The listing builds one solid part. Answer for the finished solid, in the listing's coordinates (mm). A direction names the side the tool comes from. Give positions to 0.01 mm unless a question says otherwise; leave off trailing zeros. Loops run counter-clockwise (first coordinate to the right, second up) from the corner with the lowest first, then second, coordinate; pieces in that order, holes last. Notation, with made-up numbers: M -8.75,83 L 29.25,83 A34 ccw 29.25,113 Z; hole C 40,15.25 d8. An arc over 180 degrees is marked long. One line per item, written item: value. Start each with the question number.
Q1. For faces 4 (the flat face through (39, 3, 35)), 5 (the cylindrical face through (-43.103, 2.958, 31.21)), 6 (the flat face through (-40, 3, 35)), determine the directions among +Z, -Z, +X, -X, +Y, -Y from which every point of the face is accessible in a straight line to the end or side of a thin tool.
Q2. The mould has two halves that part along Z. Classify faces 1 (the flat face through (-39, 3, -35)), 2 (the cylindrical face through (0, 3, 44)), 3 (the cylindrical face through (-0.469, 2.958, 47.498)): +Z half, -Z half, draft (parallel to the pull), parting line (faces both ways), or undercut.
Q3. Flat-ended cylindrical pins translate along their axes: pin 1 (3 mm diameter, centred on x = -37.5, y = 4, fed in from -Z); pin 2 (3 mm diameter, centred on x = -40.5, y = 4.5, fed in from +Z); pin 3 (1.5 mm diameter, centred on x = 21.5, y = 2.5, fed in from -Z). Find the tip coordinate at first contact, or state that the pin passes through.
Q4. Consider L1, parallel to X at y = 2.75, z = 0; L2, parallel to X at y = 4, z = 30; L3, parallel to Z at x = -42.5, y = 3.85. Determine where each line is inside the solid, lowest interval first.
Q5. A cutting plane is placed at C-C, the plane y = 3.5. State how many separate pieces and enclosed holes the cut face has, and give its area (3 significant figures).
Q6. A cutting plane is placed at D-D, the plane x = -17. Determine the outline of the cut face in (y, z), and give its area (3 significant figures).
Q7. A cutting plane is placed at A-A, the plane x = 0. Determine the outline of the cut face in (y, z).
Q8. A cutting plane is placed at B-B, the plane z = 12. Determine the outline of the cut face in (x, y), and give its area (3 significant figures).
from build123d import *

# Parameters (mm, degrees)
SKETCH1_R           = 2.25
SKETCH1_R_2         = 25
SKETCH1_R_3         = 1.5
BOSS_EXTRUDE1_DEPTH = 6


with BuildPart() as part:
    # Sketch1 → Boss-Extrude1 (new body)
    with BuildSketch(Plane(origin=(0, 0, 0), x_dir=(1, 0, 0), z_dir=(0, 1, 0))):
        with BuildLine():
            Line((50, -30), (50, 30))
            ThreePointArc((50, 30), (48.535533906, 33.535533906), (45, 35))
            Line((45, 35), (34.003676272, 35))
            ThreePointArc((34.003676272, 35), (32.278512373, 35.307046823), (30.765230913, 36.19047619))
            ThreePointArc((30.765230913, 36.19047619), (0, 47.5), (-30.765230913, 36.19047619))
            ThreePointArc((-30.765230913, 36.19047619), (-32.278512373, 35.307046823), (-34.003676272, 35))
            Line((-34.003676272, 35), (-45, 35))
            ThreePointArc((-45, 35), (-48.535533906, 33.535533906), (-50, 30))
            Line((-50, 30), (-50, -30))
            ThreePointArc((-50, -30), (-48.535533906, -33.535533906), (-45, -35))
            Line((-45, -35), (-34.003676272, -35))
            ThreePointArc((-34.003676272, -35), (-32.278512373, -35.307046823), (-30.765230913, -36.19047619))
            ThreePointArc((-30.765230913, -36.19047619), (0, -47.5), (30.765230913, -36.19047619))
            ThreePointArc((30.765230913, -36.19047619), (32.278512373, -35.307046823), (34.003676272, -35))
            Line((34.003676272, -35), (45, -35))
            ThreePointArc((45, -35), (48.535533906, -33.535533906), (50, -30))
        make_face()
        with Locations(Location((-45, 30, 0), (0, 0, 270))):
            Circle(SKETCH1_R, mode=Mode.SUBTRACT)
        with Locations(Location((-45, -30, 0), (0, 0, 270))):
            Circle(SKETCH1_R, mode=Mode.SUBTRACT)
        with Locations(Location((45, -30, 0), (0, 0, 270))):
            Circle(SKETCH1_R, mode=Mode.SUBTRACT)
        with Locations(Location((45, 30, 0), (0, 0, 270))):
            Circle(SKETCH1_R, mode=Mode.SUBTRACT)
        with Locations(Location((0, 0, 0), (0, 0, 270))):
            Circle(SKETCH1_R_2, mode=Mode.SUBTRACT)
        with Locations(Location((0, 42.5, 0), (0, 0, 270))):
            Circle(SKETCH1_R_3, mode=Mode.SUBTRACT)
        with Locations(Location((42.5, 0, 0), (0, 0, 270))):
            Circle(SKETCH1_R_3, mode=Mode.SUBTRACT)
        with Locations(Location((0, -42.5, 0), (0, 0, 90))):
            Circle(SKETCH1_R_3, mode=Mode.SUBTRACT)
        with Locations(Location((-42.5, 0, 0), (0, 0, 90))):
            Circle(SKETCH1_R_3, mode=Mode.SUBTRACT)
    extrude(amount=BOSS_EXTRUDE1_DEPTH)


solid = part.part
Answer block:
1. face 4: +Z, +X, +Y, -Y
1. face 5: +Y, -Y
1. face 6: +Z, -X, +Y, -Y
2. face 1: -Z half
2. face 2: undercut
2. face 3: +Z half
3. pin 1: z = -35
3. pin 2: z = 35
3. pin 3: z = -42.73
4. L1: -50 to -44, -41 to -25, 25 to 41, 44 to 50
4. L2: -50 to -47.25, -42.75 to 42.75, 47.25 to 50
4. L3: -35 to -1.5, 1.5 to 35
5. separate pieces: 1
5. enclosed holes: 9
5. area: 6,030 mm^2
6. outline: M 0,-44.35 L 6,-44.35 L 6,-18.33 L 0,-18.33 Z; M 0,18.33 L 6,18.33 L 6,44.35 L 0,44.35 Z
6. area: 312 mm^2
7. outline: M 0,-47.5 L 6,-47.5 L 6,-44 L 0,-44 Z; M 0,-41 L 6,-41 L 6,-25 L 0,-25 Z; M 0,25 L 6,25 L 6,41 L 0,41 Z; M 0,44 L 6,44 L 6,47.5 L 0,47.5 Z
8. outline: M -50,0 L -21.93,0 L -21.93,6 L -50,6 Z; M 21.93,0 L 50,0 L 50,6 L 21.93,6 Z
8. area: 337 mm^2
